Part print with two shaded views. Sizes in mm from the minimum x, y, z corner. Round coordinates to 2 decimals unless told otherwise and drop trailing zeros. Order: outer loops, then holes, each group sorted by start corner. A loop starts at its lowest first (then second) coordinate and runs counter-clockwise, first axis right, second up. Notation, with made-up numbers: (-22.5, 2) - (33.5, 2) arc R12 ccw to (33.5, 10) - close; hole circle Ø5 at (25, 48). An arc over 180 degrees is marked (long way). Answer as CSV lines item,"result". Start each with the question number.
1. Pin check, flat tips, straight feed: pin 1 Ø5 at (x, z) = (12, 82) entering from +Y; pin 2 Ø0.8 at (x, y) = (94.5, 3) entering from -Z; pin 3 Ø2 at (x, z) = (23, 58.5) entering from +Y; pin 4 Ø0.8 at (y, z) = (2.5, 64) entering from +X. Stop position of each tip, or through.
2. Band-saw the part on C-C on x = 112. List the corners of the cut face in (y, z), then the cut area to 3 significant figures.
3. Band-saw the part on A-A on z = 12. List the corners of the cut face in (x, y), then the cut area to 3 significant figures.
4. Band-saw the part on D-D on z = 33.5. List the corners of the cut face in (x, y).
5. Band-saw the part on B-B on x = 152. List the corners of the cut face in (y, z).
6. Wall check: line 1 along X through (y, z) = (0.85, 82); line 2 along Z through (x, y) = (152, 1); line 3 along Y through (x, z) = (30, 8). Give the ranges that are in metal, low to high. Write a range as [from, to].
7. Pull direction Z, two halves, no side cores. Call the marked faces 1 and 2: released by +Z, released by -Z, zero draft, split by the parting line, or undercut.
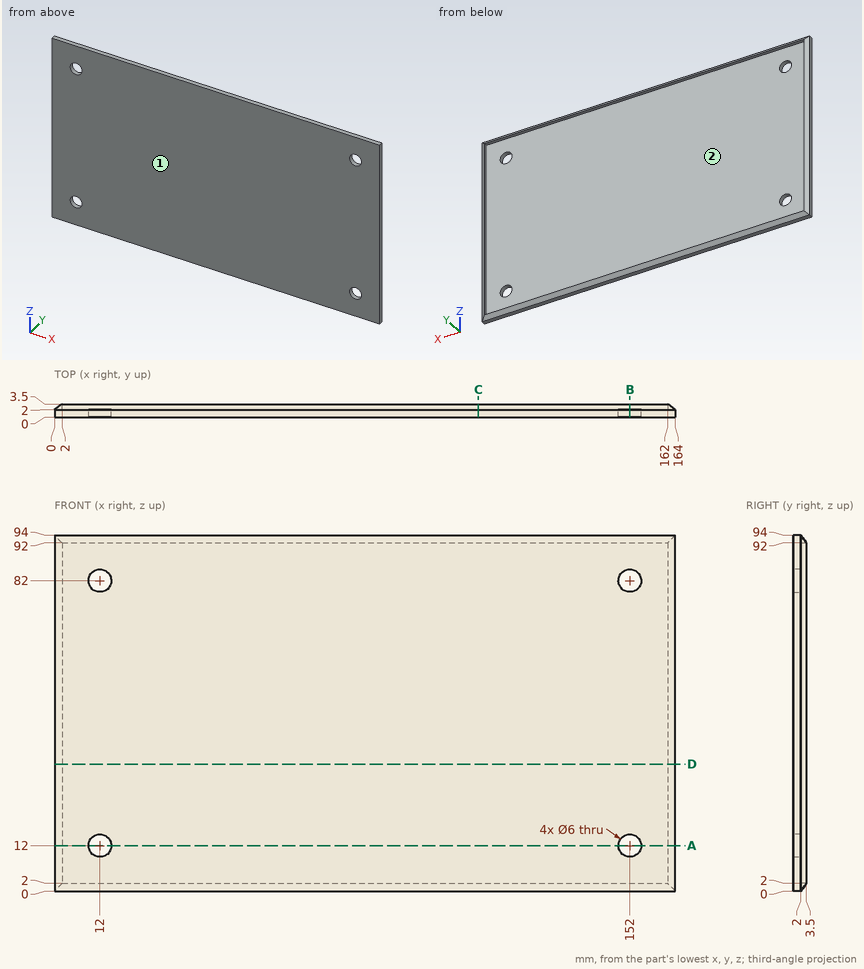
Reply:
1,pin 1,"passes through"
1,pin 2,"stops at z = 0.8"
1,pin 3,"stops at y = 2"
1,pin 4,"stops at x = 163.87"
2,outline,"(0, 0) - (2, 0) - (3.5, 2) - (2, 2) - (2, 92) - (3.5, 92) - (2, 94) - (0, 94) - close"
2,area,"191 mm2"
3,outline,"(0, 0) - (9, 0) - (9, 2) - (2, 2) - (2, 3.5) - (0, 2) - close; (15, 0) - (149, 0) - (149, 2) - (15, 2) - close; (155, 0) - (164, 0) - (164, 2) - (162, 3.5) - (162, 2) - (155, 2) - close"
3,area,"307 mm2"
4,outline,"(0, 0) - (164, 0) - (164, 2) - (162, 3.5) - (162, 2) - (2, 2) - (2, 3.5) - (0, 2) - close"
5,outline,"(0, 0) - (2, 0) - (3.5, 2) - (2, 2) - (2, 9) - (0, 9) - close; (0, 15) - (2, 15) - (2, 79) - (0, 79) - close; (0, 85) - (2, 85) - (2, 92) - (3.5, 92) - (2, 94) - (0, 94) - close"
6,line 1,"x = [0, 9], [15, 149], [155, 164]"
6,line 2,"z = [0, 9], [15, 79], [85, 94]"
6,line 3,"y = [0, 2]"
7,face 1,"zero draft"
7,face 2,"undercut"
